Read the model definition and answer for the solid it produces. Units are mm, in the model's axes. A direction names the side the tool comes from. Coordinates: 2 decimals unless noted, no trailing zeros. Loops run counter-clockwise (first coordinate to the right, second up) from the corner with the lowest first, then second, coordinate; pieces in that order, holes last.
Q1. Straight lines are drawn through the part: line 1 (X direction, y = -3.25, z = 0); line 2 (X direction, y = 1.5, z = -4); line 3 (X direction, y = -3.5, z = 5.5). For each, find the intervals that lie inside material, in ascending order.
Q2. Section D-D (y = 4) is taken. Give the vertices of the cut face in (x, z), then the cut area to 3 significant figures.
Q3. Section B-B (y = 0) is taken. Give the vertices of the cut face in (x, z).
Q4. The mould has two halves that part along X. Classify faces 1 (the face through (51.96, -3.74, -0.28)), 2 (the face through (65.811, -4, 0)), 3 (the face through (0, 0, 0)): pulls with the +X half, pulls with the -X half, needs draft (parallel to the pull), parting line crosses it, or undercut.
Q5. Which of the six approach directions +Z, -Z, +X, -X, +Y, -Y give full straight-line access (tool end or side, diameter ignored) to faces 4 (the face through (51.5, -2.504, 0.1)), 5 (the face through (51.8, -5.004, 0.1)), 6 (the face through (25.04, -1.73, 7.81))?
Q6. Flat-ended cylindrical pins translate along their axes: P1, Ø2, axis at y = 0.5, z = -3.5, coming from the +X side; P2, Ø6, axis at x = 26, y = 6.5, coming from the -Z side; P3, Ø1.9, axis at x = 62, z = 0.5, coming from the -Y side; P4, Ø2, axis at x = 10, z = 3.5, coming from the -Y side. Find the tip coordinate at first contact, or state that the pin passes through.
Q7. Section A-A (z = 0) is taken. Give the vertices of the cut face in (x, y), then the cut area to 3 significant figures.
Q8. Section C-C (x = 15) is taken. Give the vertices of the cut face in (y, z).
Autodesk Inventor part; units mm, degrees
ref_plane "YZ Plane" through (0, 0, 0) normal (1, 0, 0) x (0, 1, 0)
ref_plane "XZ Plane" through (0, 0, 0) normal (0, 1, 0) x (-1, 0, 0)
ref_plane "XY Plane" through (0, 0, 0) normal (0, 0, 1) x (1, 0, 0)
sketch "Sketch1" plane through (0, 0, 0) normal (1, 0, 0) x (0, 1, 0)
  circle A0 centre (0, 0) radius 8.001
  dimension "d0" = 16.002
extrude "Extrusion1" add sketch "Sketch1" along normal blind 50.8
sketch "Sketch2" plane through (50.8, 0, 0) normal (1, 0, 0) x (0, 0, -1)
  line L0 (-6.2432, -5.0038) -> (6.2432, -5.0038)
  line L1 (-7.5991, -2.5038) -> (7.5991, -2.5038)
  arc A0 (6.2432, -5.0038) -> (7.5991, -2.5038) centre (0, 0) ccw
  arc A1 (-7.5991, -2.5038) -> (-6.2432, -5.0038) centre (0, 0) ccw
  circle A2 centre (0, 0) radius 8.001
  point P0 (7.0332, -3.8145)
  point P1 (-7.0332, -3.8145)
  dimension "d3" = 5.0038
  dimension "d4" = 2.5
extrude "Extrusion2" add sketch "Sketch2" along normal blind 15.0114 contours A1 L1 A0 L0
sketch "Sketch3" plane through (50.8, -2.5038, 7.5991) normal (0, 1, 0) x (1, 0, 0)
  circle A0 centre (7.5057, 7.5991) radius 6.35
  line L0 (0, 15.1983) -> (15.0114, 15.1983)
  line L1 (0, 0) -> (15.0114, 0)
  point P0 (-50.8, 7.5991)
  point P1 (7.5057, 15.1983)
  dimension "d8" = 12.7
  dimension "d9" = 7.5991
  dimension "d10" = 15.1983
extrude "Extrusion3" cut sketch "Sketch3" against normal blind 15.0114
equation "\"d9\" = 0.5 * d10"
properties part number "Ring Connector model 3"
Numbers:
1. line 1: x = 0 to 51.96, 64.66 to 65.81
1. line 2: x = 0 to 50.8
1. line 3: x = 0 to 55.13, 61.48 to 65.81
2. outline: (0, -6.93) - (50.8, -6.93) - (50.8, 6.93) - (0, 6.93) - close
2. area: 704 mm2
3. outline: (0, -8) - (50.8, -8) - (50.8, 8) - (0, 8) - close
4. face 1: undercut
4. face 2: pulls with the +X half
4. face 3: pulls with the -X half
5. face 4: +Z, -Z, +X, +Y
5. face 5: +Z, -Z, +X, -Y
5. face 6: +X, -X
6. P1: stops at x = 50.8
6. P2: stops at z = -7.19
6. P3: passes through
6. P4: stops at y = -7.6
7. outline: (0, -8) - (50.8, -8) - (50.8, -5) - (51.96, -5) - (51.96, -2.5) - (50.8, -2.5) - (50.8, 8) - (0, 8) - close; (64.66, -5) - (65.81, -5) - (65.81, -2.5) - (64.66, -2.5) - close
7. area: 819 mm2
8. outline: circle Ø16 at (0, 0)
